The drawing under review shows one solid part. Ordinate dimensions are in mm from its lowest x, y, z. Coordinates: 2 decimals unless noted, no trailing zeros. Order: outer loops, then holes, each group sorted by start corner. A loop starts at its lowest first (then second) coordinate and runs counter-clockwise, first axis right, second up. Notation, with made-up numbers: (-8, -10) -> (37, -10) arc R9 ccw to (37, -1) -> close; hole circle Ø9 at (-19, 71). An arc over 180 degrees is marked (long way). Put each result on its own line as item: value.
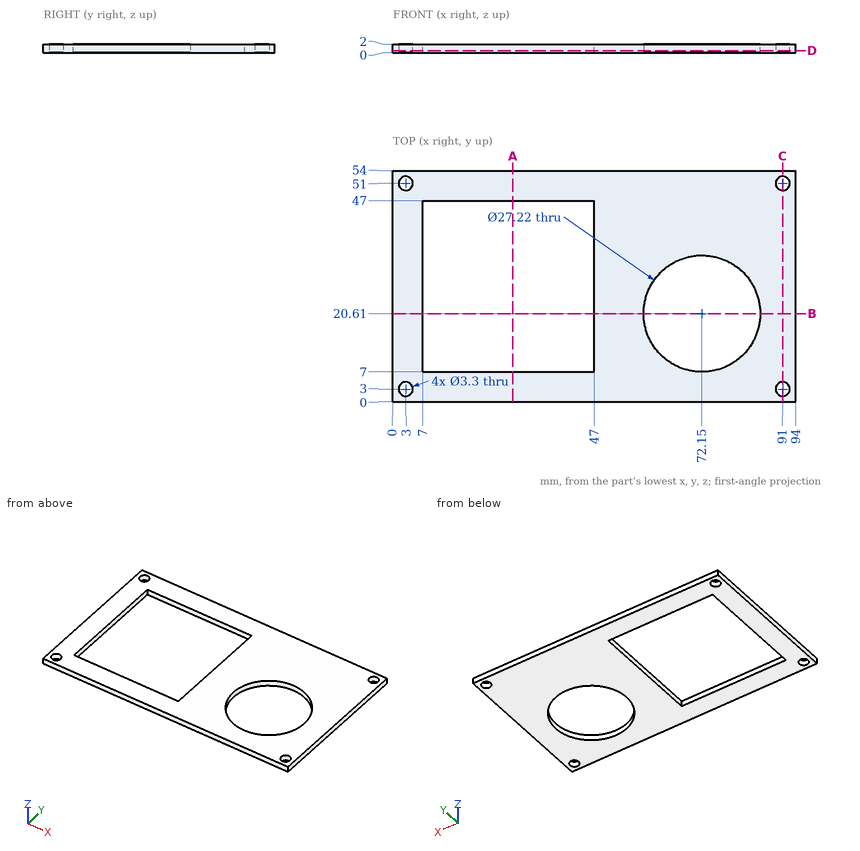
Item 1: Consider section D-D on z = 0.45. Write out the cut boundary in (x, y).
Answers below:
outline: (0, 0) -> (94, 0) -> (94, 54) -> (0, 54) -> close; hole circle Ø3.3 at (3, 3); hole circle Ø3.3 at (3, 51); hole (7, 7) -> (47, 7) -> (47, 47) -> (7, 47) -> close; hole circle Ø27.22 at (72.15, 20.61); hole circle Ø3.3 at (91, 3); hole circle Ø3.3 at (91, 51)
Item 2: For pin 1 Ø1 at (x, z) = (26, 1) entering from -Y, flat-tipped, find the tip position at first contact; note if it passes through.
Answers below:
pin 1: y = 0
Item 3: Consider section B-B on y = 20.61. Write out the cut boundary in (x, z), and give its area (3 significant figures).
Answers below:
outline: (0, 0) -> (7, 0) -> (7, 2) -> (0, 2) -> close; (47, 0) -> (58.54, 0) -> (58.54, 2) -> (47, 2) -> close; (85.76, 0) -> (94, 0) -> (94, 2) -> (85.76, 2) -> close
area: 53.6 mm^2
Item 4: Consider section C-C on x = 91. Write out the cut boundary in (y, z), and give its area (3 significant figures).
Answers below:
outline: (0, 0) -> (1.35, 0) -> (1.35, 2) -> (0, 2) -> close; (4.65, 0) -> (49.35, 0) -> (49.35, 2) -> (4.65, 2) -> close; (52.65, 0) -> (54, 0) -> (54, 2) -> (52.65, 2) -> close
area: 94.8 mm^2
Item 5: For line 1 (X direction, y = 20.61, z = 1.2); line 2 (Y direction, x = 91, z = 0.9); line 3 (X direction, y = 45, z = 0.9), list the stretches that pass through material, from the lowest coordinate up. Write a range as from..to.
Answers below:
line 1: 0..7, 47..58.54, 85.76..94
line 2: 0..1.35, 4.65..49.35, 52.65..54
line 3: 0..7, 47..94
Item 6: Consider section A-A on x = 28. Write out the cut boundary in (y, z).
Answers below:
outline: (0, 0) -> (7, 0) -> (7, 2) -> (0, 2) -> close; (47, 0) -> (54, 0) -> (54, 2) -> (47, 2) -> close
